```python
from build123d import *

# Parameters (mm, degrees)
SKETCH_1_W          = 15.5
SKETCH_1_H          = 68.5
EXTRUDE_1_DEPTH     = 150
SKETCH_2_W          = 5.5
SKETCH_2_H          = 13
CUT_EXTRUDE_1_DEPTH = 10
CHAMFER_1_SIZE      = 0.5
FILLET_1_R          = 7.5
FILLET_2_R          = 3
SKETCH_3_R          = 7.25
SKETCH_3_R_2        = 7.05
CUT_EXTRUDE_2_DEPTH = 0.5


with BuildPart() as part:
    # ｽｹｯﾁ1 → ﾎﾞｽ - 押し出し1 (new body)
    with BuildSketch(Plane(origin=(0, 0, 0), x_dir=(1, 0, 0), z_dir=(0, 1, 0))):
        Rectangle(SKETCH_1_W, SKETCH_1_H)
    extrude(amount=EXTRUDE_1_DEPTH)

    # ｽｹｯﾁ2 → ｶｯﾄ - 押し出し1 (cut)
    with BuildSketch(Plane(origin=(0, 150, 0), x_dir=(1, 0, 0), z_dir=(0, 1, 0))):
        with Locations((0, 14.75)):
            Rectangle(SKETCH_2_W, SKETCH_2_H)
        with BuildLine():
            Line((-0.75, -13.25), (0.75, -13.25))
            ThreePointArc((0.75, -13.25), (1.457106781, -13.542893219), (1.75, -14.25))
            Line((1.75, -14.25), (1.75, -21.25))
            ThreePointArc((1.75, -21.25), (1.457106781, -21.957106781), (0.75, -22.25))
            Line((0.75, -22.25), (-0.75, -22.25))
            ThreePointArc((-0.75, -22.25), (-1.457106781, -21.957106781), (-1.75, -21.25))
            Line((-1.75, -21.25), (-1.75, -14.25))
            ThreePointArc((-1.75, -14.25), (-1.457106781, -13.542893219), (-0.75, -13.25))
        make_face()
    extrude(amount=-CUT_EXTRUDE_1_DEPTH, mode=Mode.SUBTRACT)

    # 面取り1
    chamfer_1_edges = [part.edges().sort_by_distance(p)[0] for p in [
        (2.75, 150, -14.75),
        (0, 150, -21.25),
        (-2.75, 150, -14.75),
        (0, 150, -8.25),
        (1.457106781, 150, 21.957106781),
        (1.75, 150, 17.75),
        (1.457106781, 150, 13.542893219),
        (0, 150, 13.25),
        (-1.457106781, 150, 13.542893219),
        (-1.75, 150, 17.75),
        (-1.457106781, 150, 21.957106781),
        (0, 150, 22.25),
    ]]
    chamfer(chamfer_1_edges, length=CHAMFER_1_SIZE)

    # ﾌｨﾚｯﾄ1
    fillet_1_edges = [part.edges().sort_by_distance(p)[0] for p in [
        (0, 150, 34.25),
        (0, 0, 34.25),
        (0, 0, -34.25),
        (0, 150, -34.25),
    ]]
    fillet(fillet_1_edges, radius=FILLET_1_R)

    # ﾌｨﾚｯﾄ2
    fillet_2_edges = [part.edges().sort_by_distance(p)[0] for p in [
        (-7.75, 75, -34.25),
        (7.75, 75, -34.25),
        (-7.75, 0, 0),
        (-7.75, 75, 34.25),
        (-7.75, 150, 0),
        (-7.75, 147.803300859, 32.053300859),
        (-7.75, 147.803300859, -32.053300859),
        (-7.75, 2.196699141, 32.053300859),
        (-7.75, 2.196699141, -32.053300859),
        (7.75, 0, 0),
        (7.75, 150, 0),
        (7.75, 75, 34.25),
        (7.75, 147.803300859, 32.053300859),
        (7.75, 147.803300859, -32.053300859),
        (7.75, 2.196699141, 32.053300859),
        (7.75, 2.196699141, -32.053300859),
    ]]
    fillet(fillet_2_edges, radius=FILLET_2_R)

    # ｽｹｯﾁ3 → ｶｯﾄ - 押し出し2 (cut)
    with BuildSketch(Plane(origin=(7.75, 0, 0), x_dir=(0, 0, -1), z_dir=(1, 0, 0))):
        with Locations((0, 131)):
            Circle(SKETCH_3_R)
        with Locations((0, 131)):
            Circle(SKETCH_3_R_2, mode=Mode.SUBTRACT)
    extrude(amount=-CUT_EXTRUDE_2_DEPTH, mode=Mode.SUBTRACT)


solid = part.part
```
Read the model definition and answer for the solid it produces. Units are mm, in the model's axes. A direction names the side the tool comes from. Coordinates: 2 decimals unless noted, no trailing zeros. Write each loop counter-clockwise with the first axis right and the second up, starting at its lowest first coordinate (ties: lowest second). Pieces come first, ordered by that corner, then holes. Notation, with made-up numbers: (75.5, 86.25) - (98.5, 86.25) arc R10 cw to (98.5, 96.25) - close; hole circle Ø8 at (-26, -36.75). An arc over 180 degrees is marked (long way). Answer as a JSON object with one key per item and string values. Group by question number.
1. Which of the six approach directions +Z, -Z, +X, -X, +Y, -Y give full straight-line access (tool end or side, diameter ignored) to faces 1 (the flat face through (0, 140, 18)), 2 (the cylindrical face through (7.5, 138.19, 0.94)), 3 (the cylindrical face through (-6.89, 74.05, 33.35))?
2. Each of these flat-tipped pins is pushed along its axis until it touches: P1, Ø1.8, axis at x = 0, z = 19, coming from the +Y side; P2, Ø4.5, axis at x = 1, y = 146, coming from the +Z side. Where does it stop, or does it pass through?
3. A cutting plane is placed at A-A (z = -19). Determine the outline of the cut face in (x, y), plus the area to 3 significant figures.
4. Consider L1, parallel to Y at x = 7.5, z = 0; L2, parallel to Y at x = 7.4, z = 0; L3, parallel to Z at x = 5.75, y = 51. Determine where each line is inside the solid, lowest interval first. Write a range as [from, to].
5. The mould has two halves that part along Z. Classify faces 4 (the cylindrical face through (0.067, 2.255, -32.111)), 5 (the cylindrical face through (7.5, 137.99, 0.92)), 6 (the cylindrical face through (6.89, 149.1, 0.37)): +Z half, -Z half, draft (parallel to the pull), parting line (faces both ways), or undercut.
Worked out:
{
 "1": {"face 1": "+Y", "face 2": "+X", "face 3": "+Z, -X, +Y, -Y"},
 "2": {"P1": "stops at y = 140", "P2": "stops at z = 34.15"},
 "3": {"outline": "(-7.75, 3) arc R3 ccw to (-4.75, 0) - (4.75, 0) arc R3 ccw to (7.75, 3) - (7.75, 147) arc R3 ccw to (4.75, 150) - (3.25, 150) - (2.75, 149.5) - (2.75, 140) - (-2.75, 140) - (-2.75, 149.5) - (-3.25, 150) - (-4.75, 150) arc R3 ccw to (-7.75, 147) - close", "area": "2,260 mm²"},
 "4": {"L1": "y = [1.8, 123.75], [123.95, 138.05], [138.25, 148.2]", "L2": "y = [1.59, 123.75], [123.95, 138.05], [138.25, 148.41]", "L3": "z = [-34.08, 34.08]"},
 "5": {"face 4": "-Z half", "face 5": "undercut", "face 6": "draft"}
}
